Verification items for the finished model (mm, model axes). A direction names the side the tool comes from. Round coordinates to 2 decimals unless told otherwise and drop trailing zeros. Write each loop counter-clockwise with the first axis right and the second up, starting at its lowest first coordinate (ties: lowest second). Pieces come first, ordered by that corner, then holes. Notation, with made-up numbers: (50, 10) -> (92, 10) arc R17 ccw to (92, 18) -> close; hole circle Ø3 at (-6.5, 36). An arc over 180 degrees is marked (long way). Answer as a JSON object with one key per item and string values. Group by question number.
(1) Gauge pin test, flat ends, axial feed: pin 1 Ø1 at (y, z) = (50, -98.5) entering from +X; pin 2 Ø1.3 at (x, z) = (1.5, -3) entering from -Y; pin 3 Ø1.8 at (x, y) = (44, 2.5) entering from -Z. Record the tip position at first contact, or that the pin passes through.
(2) Set-up check for faces 4 (the face through (43, 74, -49)), 5 (the face through (3.5, 2, -2)), 6 (the face through (43, 2, -3.5)), 7 (the face through (41.5, 2, -98)), 8 (the face through (3.5, 2, -98)): record each of +Z, -Z, +X, -X, +Y, -Y from which the full face is reachable in a straight line by a thin tool's end or side.
(3) Draft check along Y on faces 1 (the face through (22.23, 0.9, -99.14)), 2 (the face through (22, 74, 0)), 3 (the face through (19.248, 11.357, -0.986)). Enter one of: released by +Y, released by -Y, zero draft, split by the parting line, or undercut.
(4) Sectioned sample at D-D on y = 97. Record the cut outline in (x, z), and give its area (3 significant figures).
(5) Sectioned sample at C-C on x = 22. Record the cut outline in (y, z), and give its area (3 significant figures).
(6) Sectioned sample at A-A on y = 136. Record the cut outline in (x, z), and give its area (3 significant figures).
(7) Scan lines: L1, parallel to Z at x = 10, y = 48.5; L2, parallel to X at y = 6.5, z = -84; L3, parallel to Y at x = 22, z = -99.15. Record each from-to range of solid material in increasing order. Write a range as from..to.
(8) Sectioned sample at B-B on y = 26. Record the cut outline in (x, z).
```python
from build123d import *

# Parameters (mm, degrees)
SKETCH7_W              = 45
SKETCH7_H              = 100
BOSS_EXTRUDE1_DEPTH    = 147
SHELL1_T               = -2
CONVERT_SOLID1_START   = -1
CONVERT_SOLID1_DEPTH   = 3.353553391
CONVERT_SOLID1_START_2 = 42.646446609
CONVERT_SOLID1_2_DEPTH = 3.353553391
CONVERT_SOLID1_START_3 = 2.353553391
CONVERT_SOLID1_3_DEPTH = 40.292893218
CONVERT_SOLID1_4_DEPTH = 1.146446609
CONVERT_SOLID1_START_4 = 41.5
CONVERT_SOLID1_5_DEPTH = 1.146446609
CONVERT_SOLID1_START_5 = 3.5
CONVERT_SOLID1_6_DEPTH = 38
CONVERT_SOLID1_START_6 = -96.5
CONVERT_SOLID1_7_DEPTH = 93
CONVERT_SOLID1_8_DEPTH = 93
SKETCH13_R             = 15
CUT_EXTRUDE1_DEPTH     = 10
SKETCH14_R             = 4
CUT_EXTRUDE2_DEPTH     = 10
SKETCH15_R             = 7.5
CUT_EXTRUDE3_DEPTH     = 10


with BuildPart() as part:
    # Sketch7 → Boss-Extrude1 (new body)
    with BuildSketch(Plane(origin=(0, 0, 0), x_dir=(1, 0, 0), z_dir=(0, 1, 0))):
        with Locations((22.5, 50)):
            Rectangle(SKETCH7_W, SKETCH7_H)
    extrude(amount=BOSS_EXTRUDE1_DEPTH)

    # Shell1
    shell1_openings = [part.faces().sort_by_distance(p)[0] for p in [
        (22.5, 147, -50),
    ]]
    offset(amount=SHELL1_T, openings=shell1_openings, kind=Kind.INTERSECTION)

    # Convert-Solid1: read off the stored shape, not the designer's step
    # Convert-Solid1 outline → Convert-Solid1 (cut)
    with BuildSketch(Plane.YZ.offset(CONVERT_SOLID1_START)):
        Polygon((147, -100), (147, -97.646446609), (3.5, -97.646446609), (3.5, -96.5), (0, -96.5), (0, -100), align=None)
        Polygon((147, -2.353553391), (147, 0), (0, 0), (0, -3.5), (3.5, -3.5), (3.5, -2.353553391), align=None)
    extrude(amount=CONVERT_SOLID1_DEPTH, mode=Mode.SUBTRACT)

    # Convert-Solid1 2 outline → Convert-Solid1 2 (cut)
    with BuildSketch(Plane.YZ.offset(CONVERT_SOLID1_START_2)):
        Polygon((147, -100), (147, -97.646446609), (3.5, -97.646446609), (3.5, -96.5), (0, -96.5), (0, -100), align=None)
        Polygon((147, -2.353553391), (147, 0), (0, 0), (0, -3.5), (3.5, -3.5), (3.5, -2.353553391), align=None)
    extrude(amount=CONVERT_SOLID1_2_DEPTH, mode=Mode.SUBTRACT)

    # Convert-Solid1 3 outline → Convert-Solid1 3 (cut)
    with BuildSketch(Plane.YZ.offset(CONVERT_SOLID1_START_3)):
        with BuildLine():
            ThreePointArc((3, -100), (0.878679656, -99.121320344), (0, -97))
            Line((0, -97), (0, -100))
            Line((0, -100), (3, -100))
        make_face()
        with BuildLine():
            Line((0, 0), (0, -3))
            ThreePointArc((0, -3), (0.878679656, -0.878679656), (3, 0))
            Line((3, 0), (0, 0))
        make_face()
    extrude(amount=CONVERT_SOLID1_3_DEPTH, mode=Mode.SUBTRACT)

    # Convert-Solid1 4 outline → Convert-Solid1 4 (cut)
    with BuildSketch(Plane.YZ.offset(CONVERT_SOLID1_START_3)):
        with BuildLine():
            Line((2, -98), (2, -96.5))
            Line((2, -96.5), (0, -96.5))
            Line((0, -96.5), (0, -97))
            ThreePointArc((0, -97), (0.878679656, -99.121320344), (3, -100))
            Line((3, -100), (3.5, -100))
            Line((3.5, -100), (3.5, -98))
            Line((3.5, -98), (2, -98))
        make_face()
        with BuildLine():
            Line((0, -3.5), (2, -3.5))
            Line((2, -3.5), (2, -2))
            Line((2, -2), (3.5, -2))
            Line((3.5, -2), (3.5, 0))
            Line((3.5, 0), (3, 0))
            ThreePointArc((3, 0), (0.878679656, -0.878679656), (0, -3))
            Line((0, -3), (0, -3.5))
        make_face()
    extrude(amount=CONVERT_SOLID1_4_DEPTH, mode=Mode.SUBTRACT)

    # Convert-Solid1 5 outline → Convert-Solid1 5 (cut)
    with BuildSketch(Plane.YZ.offset(CONVERT_SOLID1_START_4)):
        with BuildLine():
            Line((2, -98), (2, -96.5))
            Line((2, -96.5), (0, -96.5))
            Line((0, -96.5), (0, -97))
            ThreePointArc((0, -97), (0.878679656, -99.121320344), (3, -100))
            Line((3, -100), (3.5, -100))
            Line((3.5, -100), (3.5, -98))
            Line((3.5, -98), (2, -98))
        make_face()
        with BuildLine():
            Line((0, -3.5), (2, -3.5))
            Line((2, -3.5), (2, -2))
            Line((2, -2), (3.5, -2))
            Line((3.5, -2), (3.5, 0))
            Line((3.5, 0), (3, 0))
            ThreePointArc((3, 0), (0.878679656, -0.878679656), (0, -3))
            Line((0, -3), (0, -3.5))
        make_face()
    extrude(amount=CONVERT_SOLID1_5_DEPTH, mode=Mode.SUBTRACT)

    # Convert-Solid1 6 outline → Convert-Solid1 6 (add)
    with BuildSketch(Plane.YZ.offset(CONVERT_SOLID1_START_5)):
        with BuildLine():
            ThreePointArc((3, -98), (2.292893219, -97.707106781), (2, -97))
            Line((2, -97), (2, -98))
            Line((2, -98), (3, -98))
        make_face()
        with BuildLine():
            Line((2, -2), (2, -3))
            ThreePointArc((2, -3), (2.292893219, -2.292893219), (3, -2))
            Line((3, -2), (2, -2))
        make_face()
    extrude(amount=CONVERT_SOLID1_6_DEPTH)

    # Convert-Solid1 7 outline → Convert-Solid1 7 (cut)
    with BuildSketch(Plane.XY.offset(CONVERT_SOLID1_START_6)):
        with BuildLine():
            Line((45, 0), (45, 3))
            ThreePointArc((45, 3), (44.121320344, 0.878679656), (42, 0))
            Line((42, 0), (45, 0))
        make_face()
        with BuildLine():
            Line((0, 0), (3, 0))
            ThreePointArc((3, 0), (0.878679656, 0.878679656), (0, 3))
            Line((0, 3), (0, 0))
        make_face()
    extrude(amount=CONVERT_SOLID1_7_DEPTH, mode=Mode.SUBTRACT)

    # Convert-Solid1 8 outline → Convert-Solid1 8 (add)
    with BuildSketch(Plane.XY.offset(CONVERT_SOLID1_START_6)):
        with BuildLine():
            Line((43, 2), (43, 3))
            ThreePointArc((43, 3), (42.707106781, 2.292893219), (42, 2))
            Line((42, 2), (43, 2))
        make_face()
        with BuildLine():
            Line((2, 2), (3, 2))
            ThreePointArc((3, 2), (2.292893219, 2.292893219), (2, 3))
            Line((2, 3), (2, 2))
        make_face()
    extrude(amount=CONVERT_SOLID1_8_DEPTH)

    # Sketch13 → Cut-Extrude1 (cut)
    with BuildSketch(Plane.XY):
        with Locations((22.5, 26)):
            Circle(SKETCH13_R)
    extrude(amount=-CUT_EXTRUDE1_DEPTH, mode=Mode.SUBTRACT)

    # Sketch14 → Cut-Extrude2 (cut)
    with BuildSketch(Plane(origin=(0, 0, -100), x_dir=(-1, 0, 0), z_dir=(0, 0, -1))):
        with Locations((-22, 26)):
            Circle(SKETCH14_R)
    extrude(amount=-CUT_EXTRUDE2_DEPTH, mode=Mode.SUBTRACT)

    # Sketch15 → Cut-Extrude3 (cut)
    with BuildSketch(Plane(origin=(0, 0, -100), x_dir=(-1, 0, 0), z_dir=(0, 0, -1))):
        with Locations((-22, 97)):
            Circle(SKETCH15_R)
    extrude(amount=-CUT_EXTRUDE3_DEPTH, mode=Mode.SUBTRACT)


solid = part.part
```
Computed values:
{
 "1": {"pin 1": "x = 42.65", "pin 2": "y = 0.2", "pin 3": "z = -96.5"},
 "2": {"face 4": "+Z, -Z, +Y", "face 5": "+Z, -X, -Y", "face 6": "+Z, +X, -Y", "face 7": "-Z, +X, -Y", "face 8": "-Z, -X, -Y"},
 "3": {"face 1": "released by -Y", "face 2": "zero draft", "face 3": "undercut"},
 "4": {"outline": "(0, -97.65) -> (2, -97.65) -> (2, -2.35) -> (0, -2.35) -> close; (2.35, -100) -> (14.5, -100) -> (14.5, -98) -> (2.35, -98) -> close; (2.35, -2) -> (42.65, -2) -> (42.65, 0) -> (2.35, 0) -> close; (29.5, -100) -> (42.65, -100) -> (42.65, -98) -> (29.5, -98) -> close; (43, -97.65) -> (45, -97.65) -> (45, -2.35) -> (43, -2.35) -> close", "area": "512 mm2"},
 "5": {"outline": "(0, -97) arc R3 ccw to (3, -100) -> (22, -100) -> (22, -98) -> (3, -98) arc R1 cw to (2, -97) -> (2, -3) arc R1 cw to (3, -2) -> (11.01, -2) -> (11.01, 0) -> (3, 0) arc R3 ccw to (0, -3) -> close; (30, -100) -> (89.5, -100) -> (89.5, -98) -> (30, -98) -> close; (40.99, -2) -> (147, -2) -> (147, 0) -> (40.99, 0) -> close; (104.5, -100) -> (147, -100) -> (147, -98) -> (104.5, -98) -> close", "area": "671 mm2"},
 "6": {"outline": "(0, -97.65) -> (2, -97.65) -> (2, -2.35) -> (0, -2.35) -> close; (2.35, -100) -> (42.65, -100) -> (42.65, -98) -> (2.35, -98) -> close; (2.35, -2) -> (42.65, -2) -> (42.65, 0) -> (2.35, 0) -> close; (43, -97.65) -> (45, -97.65) -> (45, -2.35) -> (43, -2.35) -> close", "area": "542 mm2"},
 "7": {"L1": "-100..-98, -2..0", "L2": "0..2, 43..45", "L3": "0.91..22, 30..89.5, 104.5..147"},
 "8": {"outline": "(0, -97.65) -> (2, -97.65) -> (2, -2.35) -> (0, -2.35) -> close; (2.35, -100) -> (18, -100) -> (18, -98) -> (2.35, -98) -> close; (2.35, -2) -> (7.5, -2) -> (7.5, 0) -> (2.35, 0) -> close; (26, -100) -> (42.65, -100) -> (42.65, -98) -> (26, -98) -> close; (37.5, -2) -> (42.65, -2) -> (42.65, 0) -> (37.5, 0) -> close; (43, -97.65) -> (45, -97.65) -> (45, -2.35) -> (43, -2.35) -> close"}
}
